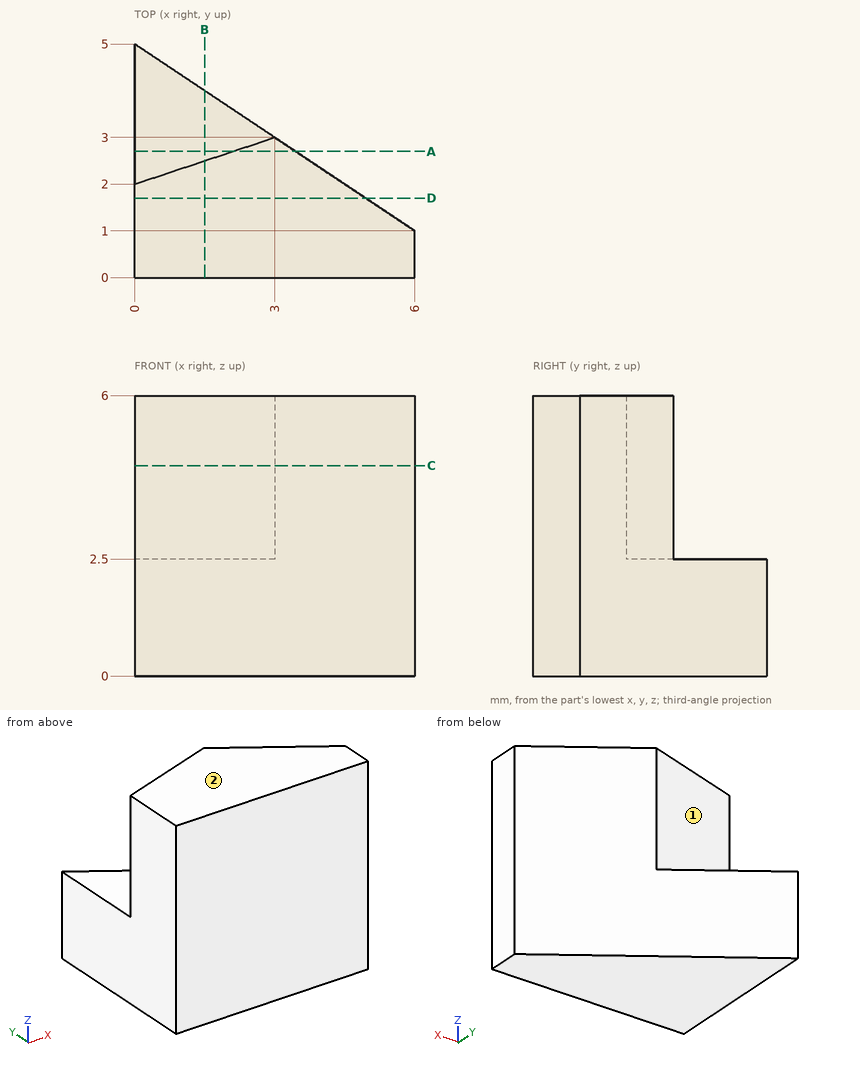
Study the drawing (mm; zero at the part's minimum x, y, z) and answer. A direction names the side the tool comes from. Coordinates: 2 decimals unless noted, no trailing zeros. Loops run counter-clockwise (first coordinate to the right, second up) from the corner with the lowest first, then second, coordinate; pieces in that order, holes last. Notation, with made-up numbers: (4, -31.5) -> (17, -31.5) arc R27 ccw to (17, 7.5) -> close; hole circle Ø11 at (72, 9). An arc over 180 degrees is marked (long way). Write each question's results on one line, items separated by ' | '. Start each with the question number.
1) Find section D-D on y = 1.7. Determine the outline of the cut face in (x, z).
2) For the marked faces 1 and 2, determine the directions among +Z, -Z, +X, -X, +Y, -Y from which every point of the face is accessible in a straight line to the end or side of a thin tool.
3) Find section C-C on z = 4.5. Determine the outline of the cut face in (x, y).
4) Find section B-B on x = 1.5. Determine the outline of the cut face in (y, z), then the cut area to 4 significant figures.
5) Consider line 1 along Y through (x, z) = (1.5, 4.7); line 2 along X through (y, z) = (1.5, 3.9). Determine where each line is inside the solid, lowest interval first.
6) Flat-ended cylindrical pins translate along their axes: P1, Ø1.5, axis at x = 1, y = 4, coming from the +Z side; P2, Ø1, axis at x = 4, z = 4, coming from the +Y side; P3, Ø1, axis at x = 3, y = 4.5, coming from the -Z side. Find the tip coordinate at first contact, or state that the pin passes through.
7) Find section A-A on y = 2.7. Determine the outline of the cut face in (x, z), then the cut area to 4 significant figures.
Response values:
1) outline: (0, 0) -> (4.95, 0) -> (4.95, 6) -> (0, 6) -> close
2) face 1: +Z, -X, +Y | face 2: +Z, +X, -X, +Y, -Y
3) outline: (0, 0) -> (6, 0) -> (6, 1) -> (3, 3) -> (0, 2) -> close
4) outline: (0, 0) -> (4, 0) -> (4, 2.5) -> (2.5, 2.5) -> (2.5, 6) -> (0, 6) -> close | area: 18.75 mm^2
5) line 1: y = 0 to 2.5 | line 2: x = 0 to 5.25
6) P1: stops at z = 2.5 | P2: stops at y = 2.67 | P3: passes through
7) outline: (0, 0) -> (3.45, 0) -> (3.45, 6) -> (2.1, 6) -> (2.1, 2.5) -> (0, 2.5) -> close | area: 13.35 mm^2
